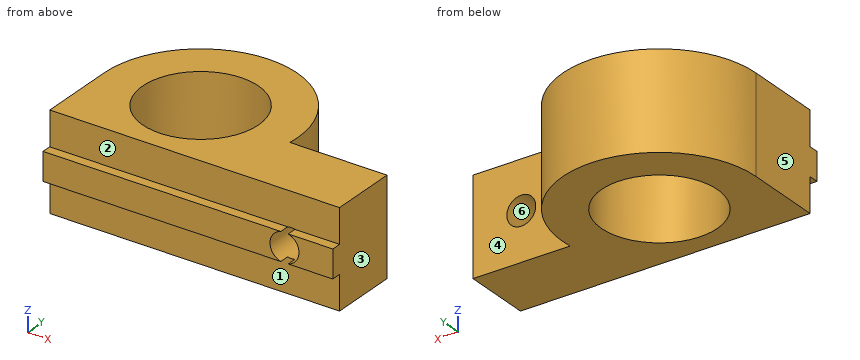
```python
from build123d import *

# Parameters (mm, degrees)
SKETCH1_R                       = 6
MAIN_DEPTH                      = 10
SKETCH3_W                       = 30
SKETCH3_H                       = 2.9
MAKERBEAMRECTANGULARGUIDE_DEPTH = 1
SKETCH4_R                       = 1.5
MAKERBEAMFIXHOLE_DEPTH          = 9


with BuildPart() as part:
    # Sketch1 → Main (new body)
    with BuildSketch(Plane.XY):
        with BuildLine():
            Line((-10, 0), (-10, -8))
            Line((-10, -8), (20, -8))
            Line((20, -8), (20, -1))
            Line((20, -1), (9.949874371, -1))
            ThreePointArc((9.949874371, -1), (0.500627751, 9.987460731), (-10, 0))
        make_face()
        Circle(SKETCH1_R, mode=Mode.SUBTRACT)
    extrude(amount=MAIN_DEPTH)

    # Sketch3 → MakerBeamRectangularGuide (add)
    with BuildSketch(Plane(origin=(0, -8, 0), x_dir=(-1, 0, 0), z_dir=(0, -1, 0))):
        with Locations((-5, -5)):
            Rectangle(SKETCH3_W, SKETCH3_H)
    extrude(amount=MAKERBEAMRECTANGULARGUIDE_DEPTH)

    # Sketch4 → MakerBeamFixHole (cut, through all)
    with BuildSketch(Plane(origin=(0, -1, 0), x_dir=(1, 0, 0), z_dir=(0, 1, 0))):
        with Locations((15, -5)):
            Circle(SKETCH4_R)
    extrude(amount=-MAKERBEAMFIXHOLE_DEPTH, mode=Mode.SUBTRACT)


solid = part.part
```
CAD build for the part. Positions are in the model's coordinates, mm. Face numbers are marked on the shaded views. A direction names the side the tool comes from. Round coordinates to 2 decimals unless told otherwise and drop trailing zeros. Order: outer loops, then holes, each group sorted by start corner. A loop starts at its lowest first (then second) coordinate and runs counter-clockwise, first axis right, second up.
Q1. Slice it at A-A (z = 5). Write the cut outline in (x, y).
Q2. Wall check: L1, parallel to Z at x = 15, y = -5.5; L2, parallel to Y at x = 0, z = 7.75; L3, parallel to X at y = -4.5, z = 5. Give the ranges that are in metal, low to high.
Q3. Slice it at B-B (x = 0). Write the cut outline in (y, z).
Q4. Drop flat-ended pins along their axis: pin 1 (4 mm diameter, centred on y = 1, z = 8, fed in from -X); pin 2 (1.1 mm diameter, centred on x = 6.5, z = 2.5, fed in from -Y); pin 3 (4 mm diameter, centred on x = 5.5, z = 6.5, fed in from +Y); pin 4 (5 mm diameter, centred on x = 16.5, z = 4.5, fed in from +Y). Give the stop position or say it passes through.
Q5. Which spindle directions (+Z, -Z, +X, -X, +Y, -Y) get a long thin tool onto all of the face, cutting with end or side? Do the marked faces 1, 2 and 3. Say none if no direction does.
Q6. Two-plate mould, pull along X, no slides. Class the marked faces 4, 5 and 6: pulls with the +X half, pulls with the -X half, needs draft (parallel to the pull), parting line crosses it, or undercut.
Q7. Slice it at C-C (y = -1.5). Write the cut outline in (x, z), and give its area (3 significant figures).
Q8. Slice it at D-D (x = 17.25). Write the cut outline in (y, z), and give its area (3 significant figures).
Results below:
1. outline: (-10, -9) - (13.5, -9) - (13.5, -1) - (9.95, -1) arc R10 ccw (long way) to (-10, 0) - close; (16.5, -9) - (20, -9) - (20, -1) - (16.5, -1) - close; hole circle Ø12 at (0, 0)
2. L1: z = 0 to 3.5, 6.5 to 10
2. L2: y = -8 to -6, 6 to 10
2. L3: x = -10 to -3.97, 3.97 to 13.5, 16.5 to 20
3. outline: (-9, 3.55) - (-8, 3.55) - (-8, 0) - (-6, 0) - (-6, 10) - (-8, 10) - (-8, 6.45) - (-9, 6.45) - close; (6, 0) - (10, 0) - (10, 10) - (6, 10) - close
4. pin 1: stops at x = -10
4. pin 2: stops at y = -8
4. pin 3: stops at y = 9.37
4. pin 4: stops at y = -1
5. face 1: -Z, +X, -X, -Y
5. face 2: +Z, +X, -X, -Y
5. face 3: +Z, -Z, +X, +Y, -Y
6. face 4: needs draft
6. face 5: pulls with the -X half
6. face 6: undercut
7. outline: (-10, 0) - (-5.81, 0) - (-5.81, 10) - (-10, 10) - close; (5.81, 0) - (20, 0) - (20, 10) - (5.81, 10) - close; hole circle Ø3 at (15, 5)
7. area: 177 mm2
8. outline: (-9, 3.55) - (-8, 3.55) - (-8, 0) - (-1, 0) - (-1, 10) - (-8, 10) - (-8, 6.45) - (-9, 6.45) - close
8. area: 72.9 mm2
